Input: part model. Units: mm. Frame: model coordinates. Face numbers are marked on the shaded views. Round coordinates to 2 decimals unless told otherwise and drop trailing zeros. Loops run counter-clockwise (first coordinate to the right, second up) from the corner with the lowest first, then second, coordinate; pieces in that order, holes last. Notation, with made-up numbers: (59.25, 65.25) - (64.25, 65.25) arc R12 ccw to (64.25, 75.25) - close; hole circle Ø8 at (31.5, 66). An arc over 180 degrees is marked (long way). Use CSV: the item, a comma, the result in double quotes. Start each with the question number.
1. Material intervals for probe 1 along Z at (x, y) = (15, 3.5); probe 2 along X at (y, z) = (1.5, -57.5); probe 3 along X at (y, z) = (2.5, -64), sorted ascending. Write a range as from..to.
2. Cut plane B-B (x = -52). Return loops of the section in (y, z), and give its area (3 significant figures).
3. Cut plane A-A (y = 5.75). Give the number of separate pieces and of enclosed holes in the cut face, and give its area (3 significant figures).
4. Pull-direction query (Y, two-part tool) for the marked faces 1 and 2; classes: +Y half, -Y half, draft (parallel to the pull), parting line (faces both ways), or undercut.
5. Pin query (flat end, axial travel): P1, Ø4, axis at x = 91, y = 7, coming from the +Z side; P2, Ø4, axis at x = -1, z = -72, coming from the +Y side; P3, Ø2, axis at x = 38, y = 5.5, coming from the +Z side; P4, Ø3, axis at y = 3.5, z = 14.5, coming from the -X side. Return the tip coordinate at first contact, or that it passes through.
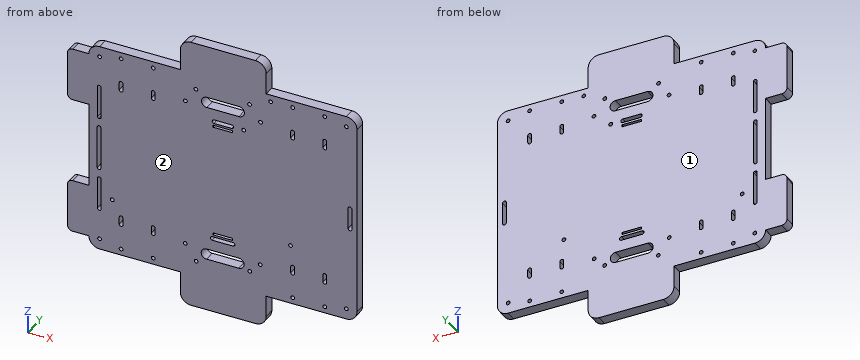
```python
from build123d import *

# Parameters (mm, degrees)
SKETCH_1_R          = 1.75
SKETCH_1_R_2        = 1.8
EXTRUDE_1_DEPTH     = 10
SKETCH_2_W          = 18.155207679
SKETCH_2_H          = 2
CUT_EXTRUDE_1_DEPTH = 10


with BuildPart() as part:
    # 草图1 → 凸台-拉伸1 (new body)
    # profile 1 of 3: a face of its own
    with BuildSketch(Plane(origin=(0, 0, 0), x_dir=(1, 0, 0), z_dir=(0, 1, 0))):
        with BuildLine():
            Line((-39.453914906, 99.953224422), (-114.8, 99.953224422))
            ThreePointArc((-114.8, 99.953224422), (-121.871067812, 97.024292234), (-124.8, 89.953224422))
            Line((-124.8, 89.953224422), (-124.8, 39.953224422))
            Line((-124.8, 39.953224422), (-124.8, -40.046775578))
            Line((-124.8, -40.046775578), (-124.8, -90.046775578))
            ThreePointArc((-124.8, -90.046775578), (-121.871067812, -97.11784339), (-114.8, -100.046775578))
            Line((-114.8, -100.046775578), (-39.453914906, -100.046775578))
            Line((-39.453914906, -100.046775578), (-39.453914906, -119.953224422))
            ThreePointArc((-39.453914906, -119.953224422), (-36.524982718, -127.024292234), (-29.453914906, -129.953224422))
            Line((-29.453914906, -129.953224422), (30.546085094, -129.953224422))
            ThreePointArc((30.546085094, -129.953224422), (37.617152905, -127.024292234), (40.546085094, -119.953224422))
            Line((40.546085094, -119.953224422), (40.546085094, -100.046775578))
            Line((40.546085094, -100.046775578), (115.2, -100.046775578))
            ThreePointArc((115.2, -100.046775578), (122.271067812, -97.11784339), (125.2, -90.046775578))
            Line((125.2, -90.046775578), (125.2, 89.953224422))
            ThreePointArc((125.2, 89.953224422), (122.271067812, 97.024292234), (115.2, 99.953224422))
            Line((115.2, 99.953224422), (40.546085094, 99.953224422))
            Line((40.546085094, 99.953224422), (40.546085094, 119.953224422))
            ThreePointArc((40.546085094, 119.953224422), (37.617152905, 127.024292234), (30.546085094, 129.953224422))
            Line((30.546085094, 129.953224422), (-29.453914906, 129.953224422))
            ThreePointArc((-29.453914906, 129.953224422), (-36.524982718, 127.024292234), (-39.453914906, 119.953224422))
            Line((-39.453914906, 119.953224422), (-39.453914906, 99.953224422))
        make_face()
        with Locations(Location((-114.8, -90.046775578, 0), (0, 0, 270))):
            Circle(SKETCH_1_R, mode=Mode.SUBTRACT)
        with Locations(Location((-94.75, -93.953224422, 0), (0, 0, 270))):
            Circle(SKETCH_1_R, mode=Mode.SUBTRACT)
        with BuildLine():
            Line((-93, -63.013616334), (-93, -69.753224422))
            ThreePointArc((-93, -69.753224422), (-94.75, -71.503224422), (-96.5, -69.753224422))
            Line((-96.5, -69.753224422), (-96.5, -63.013616334))
            ThreePointArc((-96.5, -63.013616334), (-94.75, -61.263616334), (-93, -63.013616334))
        make_face(mode=Mode.SUBTRACT)
        with Locations(Location((-64.75, -93.953224422, 0), (0, 0, 270))):
            Circle(SKETCH_1_R, mode=Mode.SUBTRACT)
        with BuildLine():
            Line((-63, -63.73712587), (-63, -69.753224422))
            ThreePointArc((-63, -69.753224422), (-64.75, -71.503224422), (-66.5, -69.753224422))
            Line((-66.5, -69.753224422), (-66.5, -63.73712587))
            ThreePointArc((-66.5, -63.73712587), (-64.75, -61.98712587), (-63, -63.73712587))
        make_face(mode=Mode.SUBTRACT)
        with Locations(Location((-25, -84.953224422, 0), (0, 0, 270))):
            Circle(SKETCH_1_R, mode=Mode.SUBTRACT)
        with Locations(Location((-34.8, -70.440823307, 0), (0, 0, 270))):
            Circle(SKETCH_1_R, mode=Mode.SUBTRACT)
        with BuildLine():
            ThreePointArc((-116.8, -30), (-116.507106781, -29.292893219), (-115.8, -29))
            Line((-115.8, -29), (-114.5, -29))
            ThreePointArc((-114.5, -29), (-113.792893219, -29.292893219), (-113.5, -30))
            Line((-113.5, -30), (-113.5, -60.81240384))
            ThreePointArc((-113.5, -60.81240384), (-115.468330013, -61.699264547), (-116.8, -60))
            Line((-116.8, -60), (-116.8, -30))
        make_face(mode=Mode.SUBTRACT)
        with BuildLine():
            Line((15.2, -79.953224422), (-14.8, -79.953224422))
            ThreePointArc((-14.8, -79.953224422), (-19.8, -74.953224422), (-14.8, -69.953224422))
            Line((-14.8, -69.953224422), (15.2, -69.953224422))
            ThreePointArc((15.2, -69.953224422), (20.2, -74.953224422), (15.2, -79.953224422))
        make_face(mode=Mode.SUBTRACT)
        with Locations(Location((25, -84.953224422, 0), (0, 0, 270))):
            Circle(SKETCH_1_R, mode=Mode.SUBTRACT)
        with Locations(Location((44.646562072, -93.418550725, 0), (0, 0, 270))):
            Circle(SKETCH_1_R, mode=Mode.SUBTRACT)
        with Locations(Location((35.2, -70.440823307, 0), (0, 0, 270))):
            Circle(SKETCH_1_R, mode=Mode.SUBTRACT)
        with Locations(Location((65.15, -93.953224422, 0), (0, 0, 270))):
            Circle(SKETCH_1_R, mode=Mode.SUBTRACT)
        with BuildLine():
            ThreePointArc((66.9, -69.753224422), (65.15, -71.503224422), (63.4, -69.753224422))
            Line((63.4, -69.753224422), (63.4, -63.73712587))
            ThreePointArc((63.4, -63.73712587), (65.15, -61.98712587), (66.9, -63.73712587))
            Line((66.9, -63.73712587), (66.9, -69.753224422))
        make_face(mode=Mode.SUBTRACT)
        with Locations(Location((95.15, -93.953224422, 0), (0, 0, 270))):
            Circle(SKETCH_1_R, mode=Mode.SUBTRACT)
        with Locations(Location((115.2, -90.046775578, 0), (0, 0, 270))):
            Circle(SKETCH_1_R, mode=Mode.SUBTRACT)
        with BuildLine():
            ThreePointArc((96.9, -69.753224422), (95.15, -71.503224422), (93.4, -69.753224422))
            Line((93.4, -69.753224422), (93.4, -63.013616334))
            ThreePointArc((93.4, -63.013616334), (95.15, -61.263616334), (96.9, -63.013616334))
            Line((96.9, -63.013616334), (96.9, -69.753224422))
        make_face(mode=Mode.SUBTRACT)
        with BuildLine():
            ThreePointArc((-8.050679844, -59.703224422), (-9.800679844, -57.953224422), (-8.050679844, -56.203224422))
            Line((-8.050679844, -56.203224422), (8.450679844, -56.203224422))
            ThreePointArc((8.450679844, -56.203224422), (10.200679844, -57.953224422), (8.450679844, -59.703224422))
            Line((8.450679844, -59.703224422), (-8.050679844, -59.703224422))
        make_face(mode=Mode.SUBTRACT)
        with Locations(Location((19.6, -57.953224422, 0), (0, 0, 270))):
            Circle(SKETCH_1_R_2, mode=Mode.SUBTRACT)
        with BuildLine():
            ThreePointArc((-116.977491453, 20), (-115.327491453, 21.65), (-113.677491453, 20))
            Line((-113.677491453, 20), (-113.677491453, -20))
            ThreePointArc((-113.677491453, -20), (-115.327491453, -21.65), (-116.977491453, -20))
            Line((-116.977491453, -20), (-116.977491453, 20))
        make_face(mode=Mode.SUBTRACT)
        with BuildLine():
            ThreePointArc((-116.8, 60), (-114.631669987, 61.699264547), (-113.5, 59.18759616))
            Line((-113.5, 59.18759616), (-113.5, 30))
            ThreePointArc((-113.5, 30), (-113.792893219, 29.292893219), (-114.5, 29))
            Line((-114.5, 29), (-115.8, 29))
            ThreePointArc((-115.8, 29), (-116.507106781, 29.292893219), (-116.8, 30))
            Line((-116.8, 30), (-116.8, 60))
        make_face(mode=Mode.SUBTRACT)
        with Locations(Location((-103, 47.79226616, 0), (0, 0, 270))):
            Circle(SKETCH_1_R_2, mode=Mode.SUBTRACT)
        with Locations(Location((-114.8, 89.953224422, 0), (0, 0, 270))):
            Circle(SKETCH_1_R, mode=Mode.SUBTRACT)
        with BuildLine():
            ThreePointArc((-96.5, 69.753224422), (-94.75, 71.503224422), (-93, 69.753224422))
            Line((-93, 69.753224422), (-93, 63.013616334))
            ThreePointArc((-93, 63.013616334), (-94.75, 61.263616334), (-96.5, 63.013616334))
            Line((-96.5, 63.013616334), (-96.5, 69.753224422))
        make_face(mode=Mode.SUBTRACT)
        with Locations(Location((-94.75, 93.953224422, 0), (0, 0, 270))):
            Circle(SKETCH_1_R, mode=Mode.SUBTRACT)
        with BuildLine():
            ThreePointArc((-66.5, 69.753224422), (-64.75, 71.503224422), (-63, 69.753224422))
            Line((-63, 69.753224422), (-63, 63.73712587))
            ThreePointArc((-63, 63.73712587), (-64.75, 61.98712587), (-66.5, 63.73712587))
            Line((-66.5, 63.73712587), (-66.5, 69.753224422))
        make_face(mode=Mode.SUBTRACT)
        with Locations(Location((-64.75, 93.953224422, 0), (0, 0, 270))):
            Circle(SKETCH_1_R, mode=Mode.SUBTRACT)
        with Locations(Location((-35, 70.440823307, 0), (0, 0, 270))):
            Circle(SKETCH_1_R, mode=Mode.SUBTRACT)
        with Locations(Location((-24.8, 84.953224422, 0), (0, 0, 270))):
            Circle(SKETCH_1_R, mode=Mode.SUBTRACT)
        with BuildLine():
            ThreePointArc((-9.793175204, 56.203224422), (-11.543175204, 57.953224422), (-9.793175204, 59.703224422))
            Line((-9.793175204, 59.703224422), (9.637810035, 59.703224422))
            ThreePointArc((9.637810035, 59.703224422), (11.387810035, 57.953224422), (9.637810035, 56.203224422))
            Line((9.637810035, 56.203224422), (-9.793175204, 56.203224422))
        make_face(mode=Mode.SUBTRACT)
        with BuildLine():
            ThreePointArc((116.858925067, 10), (118.608925067, 11.75), (120.358925067, 10))
            Line((120.358925067, 10), (120.358925067, -10))
            ThreePointArc((120.358925067, -10), (118.608925067, -11.75), (116.858925067, -10))
            Line((116.858925067, -10), (116.858925067, 10))
        make_face(mode=Mode.SUBTRACT)
        with Locations(Location((63.165136033, 43, 0), (0, 0, 270))):
            Circle(SKETCH_1_R, mode=Mode.SUBTRACT)
        with BuildLine():
            ThreePointArc((-15.044800423, 69.953224422), (-20.044800423, 74.953224422), (-15.044800423, 79.953224422))
            Line((-15.044800423, 79.953224422), (14.955199577, 79.953224422))
            ThreePointArc((14.955199577, 79.953224422), (19.955199577, 74.953224422), (14.955199577, 69.953224422))
            Line((14.955199577, 69.953224422), (-15.044800423, 69.953224422))
        make_face(mode=Mode.SUBTRACT)
        with Locations(Location((35, 70.440823307, 0), (0, 0, 270))):
            Circle(SKETCH_1_R, mode=Mode.SUBTRACT)
        with Locations(Location((25.2, 79.953224422, 0), (0, 0, 270))):
            Circle(SKETCH_1_R, mode=Mode.SUBTRACT)
        with BuildLine():
            Line((63.4, 63.73712587), (63.4, 69.753224422))
            ThreePointArc((63.4, 69.753224422), (65.15, 71.503224422), (66.9, 69.753224422))
            Line((66.9, 69.753224422), (66.9, 63.73712587))
            ThreePointArc((66.9, 63.73712587), (65.15, 61.98712587), (63.4, 63.73712587))
        make_face(mode=Mode.SUBTRACT)
        with Locations(Location((65.15, 93.953224422, 0), (0, 0, 270))):
            Circle(SKETCH_1_R, mode=Mode.SUBTRACT)
        with BuildLine():
            Line((93.4, 63.013616334), (93.4, 69.753224422))
            ThreePointArc((93.4, 69.753224422), (95.15, 71.503224422), (96.9, 69.753224422))
            Line((96.9, 69.753224422), (96.9, 63.013616334))
            ThreePointArc((96.9, 63.013616334), (95.15, 61.263616334), (93.4, 63.013616334))
        make_face(mode=Mode.SUBTRACT)
        with Locations(Location((95.15, 93.953224422, 0), (0, 0, 270))):
            Circle(SKETCH_1_R, mode=Mode.SUBTRACT)
        with Locations(Location((115.2, 89.953224422, 0), (0, 0, 270))):
            Circle(SKETCH_1_R, mode=Mode.SUBTRACT)
    # profile 2 of 3: a face of its own
    with BuildSketch(Plane(origin=(0, 0, 0), x_dir=(1, 0, 0), z_dir=(0, 1, 0))):
        with BuildLine():
            Line((-124.8, 39.953224422), (-124.8, 89.953224422))
            Line((-124.8, 89.953224422), (-139.8, 89.953224422))
            ThreePointArc((-139.8, 89.953224422), (-143.335533906, 88.488758328), (-144.8, 84.953224422))
            Line((-144.8, 84.953224422), (-144.8, 44.953224422))
            ThreePointArc((-144.8, 44.953224422), (-143.335533906, 41.417690516), (-139.8, 39.953224422))
            Line((-139.8, 39.953224422), (-124.8, 39.953224422))
        make_face()
    # profile 3 of 3: a face of its own
    with BuildSketch(Plane(origin=(0, 0, 0), x_dir=(1, 0, 0), z_dir=(0, 1, 0))):
        with BuildLine():
            Line((-124.8, -90.046775578), (-124.8, -40.046775578))
            Line((-124.8, -40.046775578), (-139.8, -40.046775578))
            ThreePointArc((-139.8, -40.046775578), (-143.335533906, -41.511241672), (-144.8, -45.046775578))
            Line((-144.8, -45.046775578), (-144.8, -85.046775578))
            ThreePointArc((-144.8, -85.046775578), (-143.335533906, -88.582309484), (-139.8, -90.046775578))
            Line((-139.8, -90.046775578), (-124.8, -90.046775578))
        make_face()
    extrude(amount=EXTRUDE_1_DEPTH)

    # 草图2 → 切除-拉伸1 (cut)
    with BuildSketch(Plane(origin=(0, 10, 0), x_dir=(1, 0, 0), z_dir=(0, 1, 0))):
        with Locations((0.054789132, -53.203224422)):
            Rectangle(SKETCH_2_W, SKETCH_2_H)
        with Locations((0.054789132, 53.203224422)):
            Rectangle(SKETCH_2_W, SKETCH_2_H)
    extrude(amount=-CUT_EXTRUDE_1_DEPTH, mode=Mode.SUBTRACT)


solid = part.part
```
Established:
1,probe 1,"z = -129.95..-79.95, -69.95..69.95, 79.95..129.95"
1,probe 2,"x = -144.8..-116.8, -113.5..-11.48, 11.33..125.2"
1,probe 3,"x = -144.8..-96.5, -93..-66.5, -63..63.4, 66.9..93.4, 96.9..125.2"
2,outline,"(0, -99.95) - (10, -99.95) - (10, 100.05) - (0, 100.05) - close"
2,area,"2,000 mm2"
3,separate pieces,"1"
3,enclosed holes,"42"
3,area,"54,700 mm2"
4,face 1,"+Y half"
4,face 2,"-Y half"
5,P1,"stops at z = 100.05"
5,P2,"passes through"
5,P3,"stops at z = 127.59"
5,P4,"stops at x = -124.8"
